Job drawing, mm, ordinate dimensions from the low corner. One solid piece. A direction names the side the tool comes from. Give positions to 0.01 mm unless a question says otherwise; leave off trailing zeros. Order: outer loops, then holes, each group sorted by start corner. A loop starts at its lowest first (then second) coordinate and runs counter-clockwise, first axis right, second up. Notation, with made-up numbers: (10, 45.25) - (47, 45.25) arc R17 cw to (47, 55.25) - close; hole circle Ø2 at (-11, -36.75). An arc over 180 degrees is marked (long way). One line per item, written item: value.
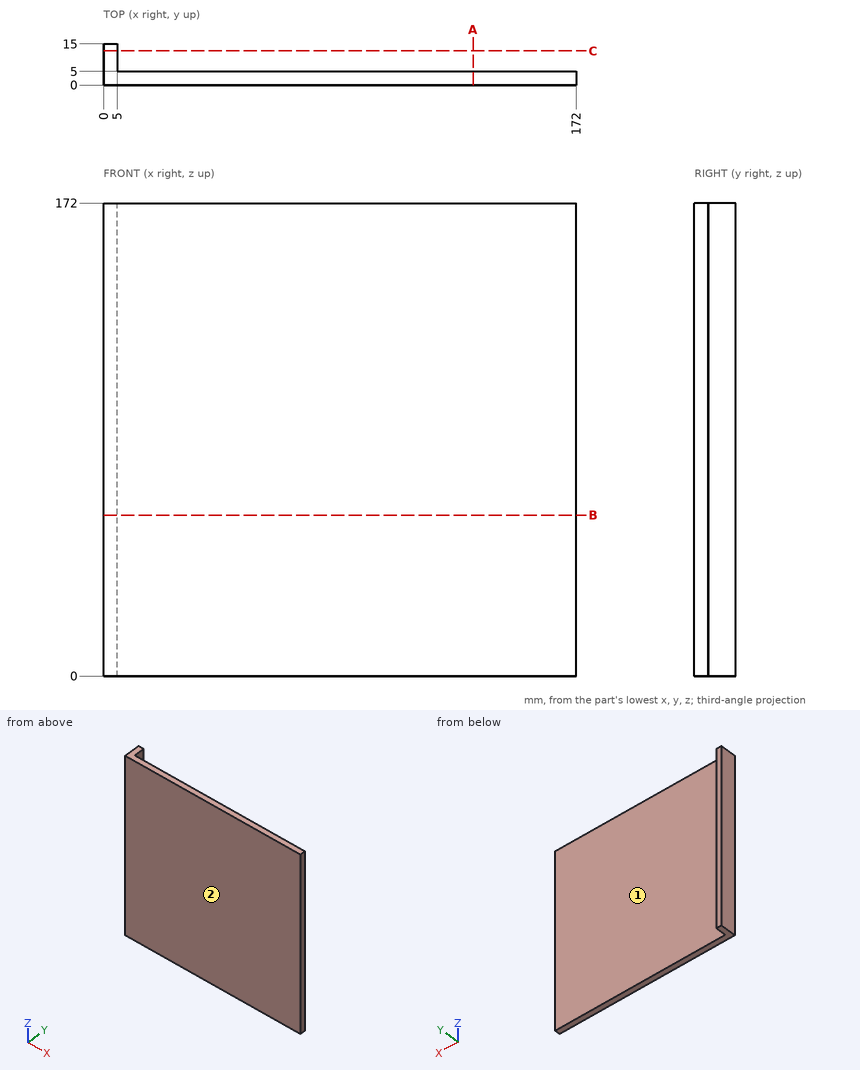
1) Drop flat-ended pins along their axis: P1, Ø1, axis at y = 5, z = 132.5, coming from the -X side; P2, Ø5, axis at x = 154, z = 94.5, coming from the +Y side; P3, Ø8, axis at y = 10.5, z = 84, coming from the +X side. Give the stop position or say it passes through.
Answer:
P1: stops at x = 0
P2: stops at y = 5
P3: stops at x = 5
2) Slice it at B-B on z = 58.5. Write the cut outline in (x, y), then the cut area to 3 significant figures.
Answer:
outline: (0, 0) - (172, 0) - (172, 5) - (5, 5) - (5, 15) - (0, 15) - close
area: 910 mm2
3) Which spindle directions (+Z, -Z, +X, -X, +Y, -Y) get a long thin tool onto all of the face, cutting with end or side? Do the marked faces 1 and 2. Say none if no direction does.
Answer:
face 1: +Z, -Z, +X, +Y
face 2: +Z, -Z, +X, -X, -Y
4) Slice it at A-A on x = 134.5. Write the cut outline in (y, z), then the cut area to 3 significant figures.
Answer:
outline: (0, 0) - (5, 0) - (5, 172) - (0, 172) - close
area: 860 mm2
5) Wall check: line 1 along X through (y, z) = (11, 28). Give the ranges that are in metal, low to high. Write a range as [from, to].
Answer:
line 1: x = [0, 5]
